CAD build for the part. Positions are in the model's coordinates, mm. Face numbers are marked on the shaded views. A direction names the side the tool comes from. Coordinates: 2 decimals unless noted, no trailing zeros. Order: outer loops, then holes, each group sorted by start corner. A loop starts at its lowest first (then second) coordinate and runs counter-clockwise, first axis right, second up. Notation, with made-up numbers: (5.25, 17.5) -> (12.25, 17.5) arc R16 ccw to (12.25, 35.5) -> close; hole circle Ø3 at (3.25, 3). An arc over 180 degrees is marked (long way). Use one line per item in the form item = value. Start each with the question number.
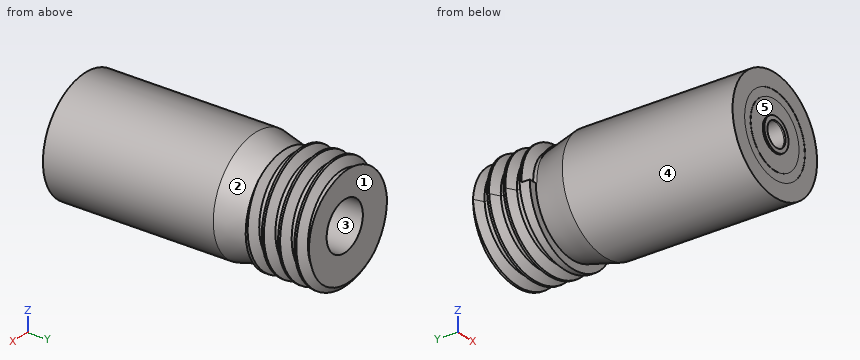
from build123d import *

# Parameters (mm, degrees)
MAINBODYS_R              = 3.5
MAIN_BODY_DEPTH          = 16
CONTACTETCHS_R           = 2.5
CONTACTETCHS_R_2         = 2
CONTACT_ETCH_DEPTH       = 0.01
ARMATURECONTACTS_R       = 1
ARMATURECONTACTS_R_2     = 0.75
ARMATURE_CONTACT_DEPTH   = 0.1
ARMATURETHRUHOLES_R      = 0.75
ARMATURE_THRU_HOLE_DEPTH = 17.748134224
BORES_R                  = 1.5
BORE_DEPTH               = 13
M7_X_5_PITCH             = 1


with BuildPart() as part:
    # MainBodyS → MAIN BODY (new body)
    with BuildSketch(Plane(origin=(0, 0, 0), x_dir=(1, 0, 0), z_dir=(0, 1, 0))):
        with Locations(Location((0, 0, 0), (0, 0, 270))):
            Circle(MAINBODYS_R)
    extrude(amount=MAIN_BODY_DEPTH)

    # ContactEtchS → CONTACT ETCH (cut)
    with BuildSketch(Plane.XZ):
        with Locations(Location((0, 0, 0), (0, 0, 270))):
            Circle(CONTACTETCHS_R)
        with Locations(Location((0, 0, 0), (0, 0, 270))):
            Circle(CONTACTETCHS_R_2, mode=Mode.SUBTRACT)
    extrude(amount=-CONTACT_ETCH_DEPTH, mode=Mode.SUBTRACT)

    # ArmatureContactS → ARMATURE CONTACT (add)
    with BuildSketch(Plane(origin=(0, 0, 0), x_dir=(-1, 0, 0), z_dir=(0, -1, 0))):
        with Locations(Location((0, 0, 0), (0, 0, 270))):
            Circle(ARMATURECONTACTS_R)
        with Locations(Location((0, 0, 0), (0, 0, 90))):
            Circle(ARMATURECONTACTS_R_2, mode=Mode.SUBTRACT)
    extrude(amount=ARMATURE_CONTACT_DEPTH)

    # ArmatureThruHoleS → ARMATURE THRU HOLE (cut, through all)
    with BuildSketch(Plane.XZ):
        with Locations(Location((0, 0, 0), (0, 0, 270))):
            Circle(ARMATURETHRUHOLES_R)
    extrude(amount=-ARMATURE_THRU_HOLE_DEPTH, mode=Mode.SUBTRACT)

    # ThreadCutS → THREAD CUT (revolve, cut)
    with BuildSketch(Plane.XY, mode=Mode.PRIVATE) as thread_cut_sk:
        Polygon((3, 12.5), (3.5, 10.5), (3.5, 12.5), align=None)
    revolve(thread_cut_sk.sketch.rotate(Axis((0, 0, 0), (0, 1, 0)), 90), axis=Axis((0, 0, 0), (0, 1, 0)), mode=Mode.SUBTRACT)

    # BoreS → BORE (cut)
    with BuildSketch(Plane(origin=(0, 16, 0), x_dir=(1, 0, 0), z_dir=(0, 1, 0))):
        with Locations(Location((0, 0, 0), (0, 0, 270))):
            Circle(BORES_R)
    extrude(amount=-BORE_DEPTH, mode=Mode.SUBTRACT)

    # M7 x .5: arcs per turn and ends read off the stored shape
    # M7 x .5: the profile of Thread Profile3 profile screwed along a right-hand helix through 4 turns, 8 arcs to a turn; built about Z, then put on its axis
    m7_x_5_z = Axis((0, 0, 0), (0, 0, 1))
    m7_x_5_corners = [(3.5003, 0, -0.000173205), (3.5003, 0, 0.875173202), (2.958734125, 0, 0.562499999), (2.958734125, 0, 0.312499999)]
    with BuildLine(mode=Mode.PRIVATE) as m7_x_5_profile:
        Line(m7_x_5_corners[0], m7_x_5_corners[1])
        Line(m7_x_5_corners[1], m7_x_5_corners[2])
        Line(m7_x_5_corners[2], m7_x_5_corners[3])
        Line(m7_x_5_corners[3], m7_x_5_corners[0])
    m7_x_5_cap = Face(m7_x_5_profile.wire())
    m7_x_5_turn_angles = [0, 22.5, 45, 67.5, 90, 112.5, 135, 157.5, 180, 202.5, 225, 247.5, 270, 292.5, 315, 337.5, 360]
    m7_x_5_turn_weights = [1, 0.9238795325112867, 1, 0.9238795325112867, 1, 0.9238795325112867, 1, 0.9238795325112867, 1, 0.9238795325112867, 1, 0.9238795325112867, 1, 0.9238795325112867, 1, 0.9238795325112867, 1]
    m7_x_5_turn_rails = [Edge.make_bspline([Vector(p[0], p[1], 0).rotate(m7_x_5_z, m7_x_5_turn_angles[k]) / m7_x_5_turn_weights[k] + Vector(0, 0, p[2] + M7_X_5_PITCH * m7_x_5_turn_angles[k] / 360) for k in range(17)], [0, 0, 0, 1, 1, 2, 2, 3, 3, 4, 4, 5, 5, 6, 6, 7, 7, 8, 8, 8], 2, m7_x_5_turn_weights) for p in m7_x_5_corners]
    m7_x_5_turn_sides = [Face.make_surface_from_curves(m7_x_5_turn_rails[p[0]], m7_x_5_turn_rails[p[1]]) for p in [(0, 1), (1, 2), (2, 3), (3, 0)]]
    m7_x_5 = Plane(origin=(0, 17, 0), x_dir=(-1, 0, 0), z_dir=(0, -1, 0)) * Solid(Shell([*[p.moved(Location((0, 0, M7_X_5_PITCH * i))) for i in range(4) for p in m7_x_5_turn_sides], m7_x_5_cap, m7_x_5_cap.rotate(m7_x_5_z, 1440).moved(Location((0, 0, M7_X_5_PITCH * 1440 / 360)))]))
    add(m7_x_5, mode=Mode.SUBTRACT)


solid = part.part
1) Cut at B-B on x = 3.25. Count the separate pieces of the cut face and the enclosed holes in it, then the cut area to 3 significant figures.
2) Cut at C-C on y = 7.5. Give the cut face in (x, z), then the cut area to 3 significant figures.
3) Cut at A-A on y = 1. Give the cut face in (x, z), then the cut area to 3 significant figures.
4) Two-plate mould, pull along Y, no slides. Class the marked faces 1, 2 and 3: released by +Y, released by -Y, zero draft, split by the parting line, or undercut.
5) Probe L1, parallel to X at y = 1.85, z = 0; L2, parallel to Y at x = 1, z = 1.5; L3, parallel to Z at x = 0.5, y = 5. List the from-to ranges inside material, lowest first.
6) 3-axis set-ups, long thin cutter, end or side, ignore diameter. For the marked faces 4 and 5: which of +Z, -Z, +X, -X, +Y, -Y reach the whole face in a straight line?
7) Drop flat-ended pins along their axis: P1, Ø4, axis at y = 3.5, z = 2.5, coming from the +X side; P2, Ø2, axis at x = 0, z = -2.5, coming from the -Y side; P3, Ø0.6, axis at x = -3.5, y = 12.5, coming from the +Z side. Give the stop position or say it passes through.
Values follow:
q1.separate_pieces = 5
q1.enclosed_holes = 0
q1.area = 32.0 mm^2
q2.outline = circle Ø7 at (0, 0); hole circle Ø3 at (0, 0)
q2.area = 31.4 mm^2
q3.outline = circle Ø7 at (0, 0); hole circle Ø1.5 at (0, 0)
q3.area = 36.7 mm^2
q4.face_1 = released by +Y
q4.face_2 = undercut
q4.face_3 = zero draft
q5.L1 = -3.5 to -0.75, 0.75 to 3.5
q5.L2 = 0 to 16
q5.L3 = -3.46 to -1.41, 1.41 to 3.46
q6.face_4 = +Y, -Y
q6.face_5 = -Y
q7.P1 = 3.46
q7.P2 = 0
q7.P3 = 0
